```python
from build123d import *

# Parameters (mm, degrees)
F2_SIZE = 0.5
F3_SIZE = 0.25


with BuildPart() as f1:
    # F0 (on Right) → F1 (revolve)
    with BuildSketch(Plane.YZ):
        Polygon((-15.9592820017, -2.8064947682), (-10.4592820017, -2.8064947682), (-10.4592820017, -0.8064947682), (-22.4592820017, -0.8064947682), (-22.4592820017, -3.8364947682), (-28.9592820017, -3.8364947682), (-28.9592820017, -5.3064947682), (-17.4592820017, -5.3064947682), (-17.4592820017, -4.3064947682), (-15.9592820017, -4.3064947682), align=None)
    revolve(axis=Axis((0, -19.7092820017, -5.4264947682), (0, 1, 0)))

    # F2
    f2_edges = [f1.edges().sort_by_distance(p)[0] for p in [
        (0, -28.959282, -7.016495),
        (0, -28.959282, -5.546495),
    ]]
    chamfer(f2_edges, length=F2_SIZE)

    # F3
    f3_edges = [f1.edges().sort_by_distance(p)[0] for p in [
        (0, -15.959282, -6.546495),
        (0, -10.459282, -8.046495),
        (0, -17.459282, -5.546495),
    ]]
    chamfer(f3_edges, length=F3_SIZE)


solid = f1.part
```
Source: CAD feature listing. Evaluate the final solid. Frame: model axes, mm. A direction names the side the tool comes from. Round coordinates to 2 decimals unless told otherwise and drop trailing zeros. Order: outer loops, then holes, each group sorted by start corner. A loop starts at its lowest first (then second) coordinate and runs counter-clockwise, first axis right, second up. Notation, with made-up numbers: (9.25, 83.25) -> (21.25, 83.25) arc R32 cw to (21.25, 115.25) -> close; hole circle Ø3 at (23, 18.25). An arc over 180 degrees is marked (long way). One line per item, written item: value. Start each with the question number.
Q1. Section query B-B (z = -8.75). Return the cut outline in (x, y), plus the area to 3 significant figures.
Q2. Section query D-D (z = -1.5). Return the cut outline in (x, y), plus the area to 3 significant figures.
Q3. Section query C-C (y = -26.25). Return the cut outline in (x, z), plus the area to 3 significant figures.
Q4. Section query A-A (y = -12). Return the cut outline in (x, z).
Q5. Draft query along Z for faces 1 (the cylindrical face through (-0.967, -25.501, -6.688)), 2 (the flat face through (0, -17.459, -6)), 3 (the flat face through (-2, -22.459, -5)). Return one class per face: pulls with the +Z half, pulls with the -Z half, needs draft (parallel to the pull), parting line crosses it, or undercut.
Q6. Material intervals for probe 1 along Y at (x, z) = (-3, -7.5); probe 2 along Y at (x, z) = (-2, -5.75); probe 3 along X at (y, z) = (-20, -5.5), sorted ascending.
Q7. Access query for faces 4 (the flat face through (-2, -10.459, -3)), 5 (the flat face through (-1, -15.959, -7)). Directions: +Z, -Z, +X, -X, +Y, -Y. A direction counts if a zero-diameter tool reaches every point of the face in a straight line with its end or side. Return the directions, or none.
Q8. Pin query (flat end, axial travel): pin 1 (1.5 mm diameter, centred on y = -27, z = -4.5, fed in from -X); pin 2 (1.8 mm diameter, centred on x = 0, z = -5.43, fed in from -Y); pin 3 (2 mm diameter, centred on x = -2, y = -15.5, fed in from -Z); pin 4 (1.5 mm diameter, centred on x = -2, z = -5.5, fed in from -Y). Return the tip coordinate at first contact, or that it passes through.
Findings below:
1. outline: (-3.21, -22.46) -> (3.21, -22.46) -> (3.21, -10.46) -> (-3.21, -10.46) -> close
1. area: 77.0 mm²
2. outline: (-2.43, -22.46) -> (2.43, -22.46) -> (2.43, -10.46) -> (-2.43, -10.46) -> close
2. area: 58.4 mm²
3. outline: circle Ø3.18 at (0, -5.43); hole circle Ø0.24 at (0, -5.43)
3. area: 7.90 mm²
4. outline: circle Ø9.24 at (0, -5.43); hole circle Ø5.24 at (0, -5.43)
5. face 1: parting line crosses it
5. face 2: undercut
5. face 3: needs draft
6. probe 1: -22.46 to -10.46
6. probe 2: -22.46 to -15.96
6. probe 3: -4.62 to -0.09, 0.09 to 4.62
7. face 4: +Z, -Z, +X, -X, +Y
7. face 5: +Y
8. pin 1: x = -1.58
8. pin 2: y = -28.96
8. pin 3: z = -9.94
8. pin 4: y = -28.8
